Job drawing, mm, ordinate dimensions from the low corner. One solid piece. A direction names the side the tool comes from. Coordinates: 2 decimals unless noted, no trailing zeros. Order: outer loops, then holes, each group sorted by start corner. A loop starts at its lowest first (then second) coordinate and runs counter-clockwise, first axis right, second up. Notation, with made-up numbers: (68.5, -6.5) - (103.5, -6.5) arc R12 cw to (103.5, 16.5) - close; hole circle Ø10 at (78.5, 33.5). An arc over 180 degrees is marked (long way). Use a Markdown table: item, result. Add a question column.
1) Saw through at C-C on y = 6.75. List the corners of the cut face in (x, z).
2) Wall check: L1, parallel to Z at x = 16.5, y = 13.5; L2, parallel to Y at x = 20.5, z = 19.5. Give the ranges that are in metal, low to high. Write a range as [from, to].
3) Two-plate mould, pull along Z, no slides. Class the marked faces 3, 4 and 5: +Z half, -Z half, draft (parallel to the pull), parting line (faces both ways), or undercut.
4) Tool access for the marked faces 1 and 2: list every direction of +Z, -Z, +X, -X, +Y, -Y with a clear straight run to the whole face (end or side of a thin tool).
5) Saw through at A-A on x = 16.5. List the corners of the cut face in (y, z), then the cut area to 3 significant figures.
6) Saw through at D-D on x = 8. List the corners of the cut face in (y, z).
7) Saw through at B-B on z = 16.5. List the corners of the cut face in (x, y), then the cut area to 3 significant figures.
8) Drop flat-ended pins along their axis: P1, Ø1, axis at x = 7.5, z = 25, coming from the +Y side; P2, Ø2, axis at y = 14, z = 9.5, coming from the -X side; P3, Ø4, axis at y = 4, z = 4.5, coming from the -X side. Give the stop position or say it passes through.
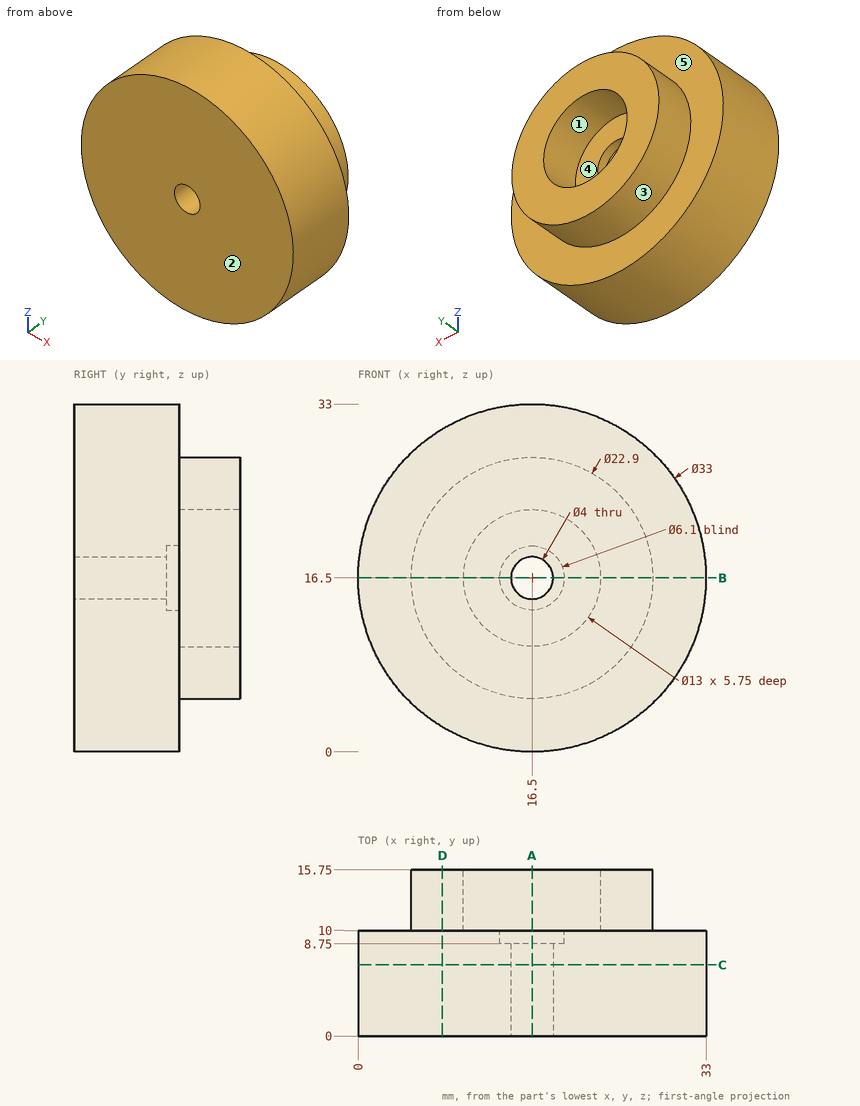
Results are:
| question | item | result |
|---|---|---|
| 1 | outline | circle Ø33 at (16.5, 16.5); hole circle Ø4 at (16.5, 16.5) |
| 2 | L1 | [5.05, 10], [23, 27.95] |
| 2 | L2 | [0, 10] |
| 3 | face 3 | parting line |
| 3 | face 4 | undercut |
| 3 | face 5 | draft |
| 4 | face 1 | +Y |
| 4 | face 2 | +Z, -Z, +X, -X, -Y |
| 5 | outline | (0, 0) - (10, 0) - (10, 5.05) - (15.75, 5.05) - (15.75, 10) - (10, 10) - (10, 13.45) - (8.75, 13.45) - (8.75, 14.5) - (0, 14.5) - close; (0, 18.5) - (8.75, 18.5) - (8.75, 19.55) - (10, 19.55) - (10, 23) - (15.75, 23) - (15.75, 27.95) - (10, 27.95) - (10, 33) - (0, 33) - close |
| 5 | area | 344 mm2 |
| 6 | outline | (0, 2.36) - (10, 2.36) - (10, 8.83) - (15.75, 8.83) - (15.75, 24.17) - (10, 24.17) - (10, 30.64) - (0, 30.64) - close |
| 7 | outline | (0, 0) - (14.5, 0) - (14.5, 8.75) - (13.45, 8.75) - (13.45, 10) - (10, 10) - (10, 15.75) - (5.05, 15.75) - (5.05, 10) - (0, 10) - close; (18.5, 0) - (33, 0) - (33, 10) - (27.95, 10) - (27.95, 15.75) - (23, 15.75) - (23, 10) - (19.55, 10) - (19.55, 8.75) - (18.5, 8.75) - close |
| 7 | area | 344 mm2 |
| 8 | P1 | y = 10 |
| 8 | P2 | x = 6.75 |
| 8 | P3 | x = 3.38 |
